Drawing for the job (mm, zero at the part's lowest x, y, z). A direction names the side the tool comes from. Coordinates: 2 decimals unless noted, no trailing zeros. Write each loop counter-clockwise with the first axis right and the second up, starting at its lowest first coordinate (ties: lowest second). Pieces come first, ordered by that corner, then holes. Notation, with made-up numbers: (26.5, 57) -> (34.5, 57) arc R24 ccw to (34.5, 67) -> close; hole circle Ø7 at (26, 54). An arc over 180 degrees is marked (long way). Write item = value, one per line. Start each with the question number.
Q1. Probe line 1 (Y direction, x = 37.5, z = 10.25); line 2 (X direction, y = 25, z = 5); line 3 (X direction, y = 32, z = 10). List the from-to ranges inside material, lowest first.
Q2. Band-saw the part on A-A, the plane z = 4.75. List the corners of the cut face in (x, y).
Q3. Pull direction Y, two halves, no side cores. Call the marked faces 1, 2, 3 and 4: released by +Y, released by -Y, zero draft, split by the parting line, or undercut.
Q4. Band-saw the part on D-D, the plane y = 20. List the corners of the cut face in (x, z), plus the area to 3 significant figures.
Q5. Band-saw the part on C-C, the plane x = 19. List the corners of the cut face in (y, z), plus the area to 3 significant figures.
Q6. Tool access for the marked faces 5 and 6: list every direction of +Z, -Z, +X, -X, +Y, -Y with a clear straight run to the whole face (end or side of a thin tool).
Q7. Band-saw the part on B-B, the plane y = 3.5. List the corners of the cut face in (x, z).
Q8. Pin check, flat tips, straight feed: P1, Ø1, axis at x = 1.5, z = 9, coming from the +Y side; P2, Ø5.5, axis at x = 4.5, y = 35.5, coming from the -Z side (3 decimals). Stop position of each tip, or through.
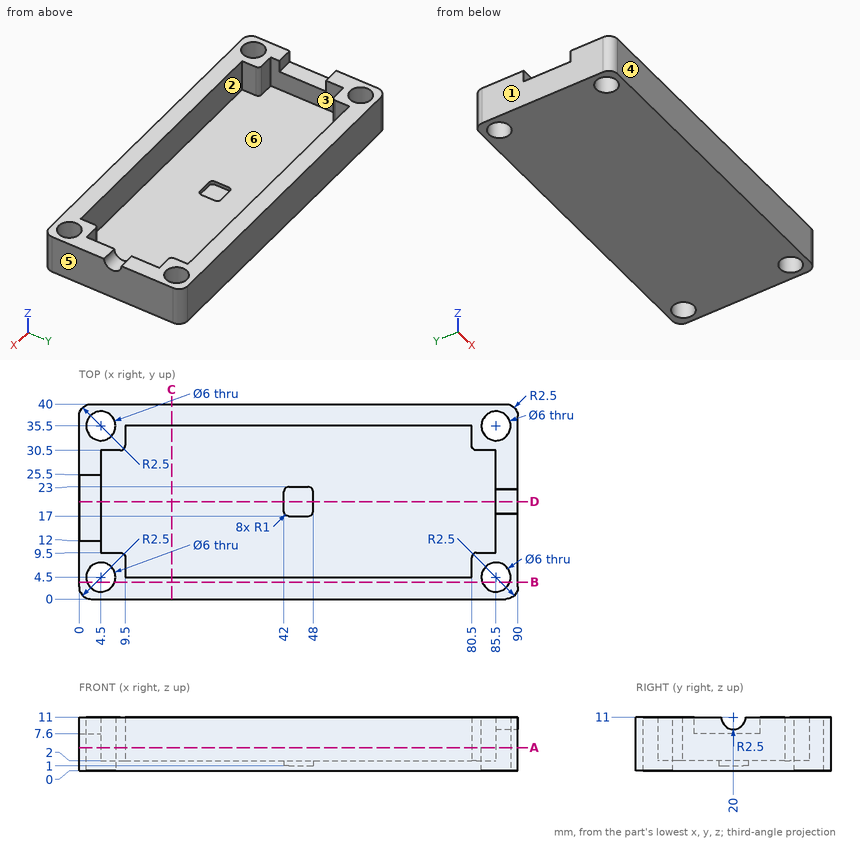
Ans:
q1.line_1 = 0 to 4.5, 35.5 to 40
q1.line_2 = 0 to 4.5, 85.5 to 90
q1.line_3 = 0 to 9.5, 80.5 to 90
q2.outline = (0, 2.5) arc R2.5 ccw to (2.5, 0) -> (87.5, 0) arc R2.5 ccw to (90, 2.5) -> (90, 37.5) arc R2.5 ccw to (87.5, 40) -> (2.5, 40) arc R2.5 ccw to (0, 37.5) -> close; hole circle Ø6 at (4.5, 4.5); hole circle Ø6 at (4.5, 35.5); hole (4.5, 9.5) -> (8.5, 9.5) arc R1 cw to (9.5, 8.5) -> (9.5, 4.5) -> (80.5, 4.5) -> (80.5, 8.5) arc R1 cw to (81.5, 9.5) -> (85.5, 9.5) -> (85.5, 30.5) -> (81.5, 30.5) arc R1 cw to (80.5, 31.5) -> (80.5, 35.5) -> (9.5, 35.5) -> (9.5, 31.5) arc R1 cw to (8.5, 30.5) -> (4.5, 30.5) -> close; hole circle Ø6 at (85.5, 4.5); hole circle Ø6 at (85.5, 35.5)
q3.face_1 = zero draft
q3.face_2 = undercut
q3.face_3 = undercut
q3.face_4 = released by -Y
q4.outline = (0, 0) -> (90, 0) -> (90, 8.5) -> (85.5, 8.5) -> (85.5, 2) -> (48, 2) -> (48, 1) -> (42, 1) -> (42, 2) -> (4.5, 2) -> (4.5, 7.6) -> (0, 7.6) -> close
q4.area = 228 mm2
q5.outline = (0, 0) -> (40, 0) -> (40, 11) -> (35.5, 11) -> (35.5, 2) -> (4.5, 2) -> (4.5, 11) -> (0, 11) -> close
q5.area = 161 mm2
q6.face_5 = +Z, -Z, +X, +Y, -Y
q6.face_6 = +Z
q7.outline = (0, 0) -> (1.67, 0) -> (1.67, 11) -> (0, 11) -> close; (7.33, 0) -> (82.67, 0) -> (82.67, 11) -> (7.33, 11) -> close; (88.33, 0) -> (90, 0) -> (90, 11) -> (88.33, 11) -> close
q8.P1 = 39.95
q8.P2 = through
